```python
from build123d import *

# Parameters (mm, degrees)
EXTRUDE_1_DEPTH     = 90.5
SKETCH_2_W          = 81.5
SKETCH_2_H          = 84
CUT_EXTRUDE_1_DEPTH = 0.6
SKETCH_3_W          = 3.2
SKETCH_3_H          = 23
CUT_EXTRUDE_2_DEPTH = 0.6


with BuildPart() as part:
    # 草图1 → 凸台-拉伸1 (new body)
    with BuildSketch(Plane(origin=(0, 0, 0), x_dir=(0, 0, -1), z_dir=(1, 0, 0))):
        Polygon((0, 0), (0, -15.1), (-112, -11), (-112, 0), align=None)
    extrude(amount=EXTRUDE_1_DEPTH)

    # 草图2 → 切除-拉伸1 (cut)
    with BuildSketch(Plane(origin=(0, 0, 0), x_dir=(1, 0, 0), z_dir=(0, 1, 0))):
        with Locations((45.25, -63)):
            Rectangle(SKETCH_2_W, SKETCH_2_H)
    extrude(amount=-CUT_EXTRUDE_1_DEPTH, mode=Mode.SUBTRACT)

    # 草图3 → 切除-拉伸2 (cut)
    with BuildSketch(Plane(origin=(0, 0, 0), x_dir=(1, 0, 0), z_dir=(0, 1, 0))):
        with Locations((86.9, -100.5)):
            Rectangle(SKETCH_3_W, SKETCH_3_H)
    extrude(amount=-CUT_EXTRUDE_2_DEPTH, mode=Mode.SUBTRACT)


solid = part.part
```
Check sheet for the modelled part. Datum: model origin and axes. Units: mm. Round coordinates to 2 decimals unless told otherwise and drop trailing zeros. Write each loop counter-clockwise with the first axis right and the second up, starting at its lowest first coordinate (ties: lowest second). Pieces come first, ordered by that corner, then holes. Notation, with made-up numbers: (10, -21.5) -> (64, -21.5) arc R16 cw to (64, -0.5) -> close; hole circle Ø6 at (-4.5, 27.5). An arc over 180 degrees is marked (long way). Put each result on its own line as item: value.
(1) Mould release check, pull along X, two halves, no side actions. Record for faces 1 (the face through (90.5, -6, 55)), 2 (the face through (35, 0, 19)), 3 (the face through (46, -0.6, 56)): released by +X, released by -X, zero draft, split by the parting line, or undercut.
Values found:
face 1: released by +X
face 2: zero draft
face 3: undercut
(2) Go/stop test with flat-tipped pins: pin 1 Ø10 at (x, z) = (36.5, 40) entering from -Y; pin 2 Ø8 at (x, z) = (65.5, 39) entering from +Y. Record where each tip stops, or that it passes through.
Values found:
pin 1: stops at y = -13.82
pin 2: stops at y = -0.6
(3) Sectioned sample at A-A (x = 13). Enter the section's corners in (y, z), plus the area to 3 significant figures.
Values found:
outline: (-15.1, 0) -> (0, 0) -> (0, 21) -> (-0.6, 21) -> (-0.6, 105) -> (0, 105) -> (0, 112) -> (-11, 112) -> close
area: 1,410 mm^2
(4) Material ranges on line 1 (Y direction, x = 75, z = 44); line 2 (Y direction, x = 35.5, z = 26), recorded low to high.
Values found:
line 1: y = -13.49 to -0.6
line 2: y = -14.15 to -0.6
(5) Sectioned sample at C-C (z = 10.5). Enter the section's corners in (x, y), plus the area to 3 significant figures.
Values found:
outline: (0, -14.72) -> (90.5, -14.72) -> (90.5, 0) -> (0, 0) -> close
area: 1,330 mm^2
(6) Sectioned sample at B-B (z = 47.5). Enter the section's corners in (x, y).
Values found:
outline: (0, -13.36) -> (90.5, -13.36) -> (90.5, 0) -> (86, 0) -> (86, -0.6) -> (4.5, -0.6) -> (4.5, 0) -> (0, 0) -> close
